Here's how the part is built. I have some questions about the finished solid (model axes, mm). Face numbers are marked on the shaded views. A direction names the side the tool comes from. Give positions to 0.01 mm unless a question says otherwise; leave off trailing zeros. Order: outer loops, then holes, each group sorted by start corner. A loop starts at its lowest first (then second) coordinate and runs counter-clockwise, first axis right, second up.
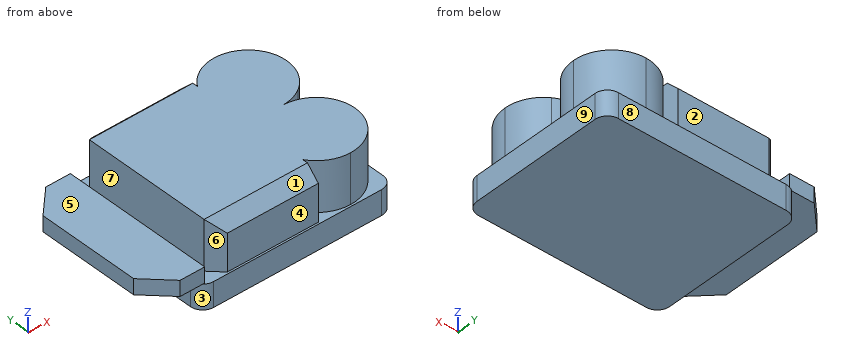
from build123d import *

# Parameters (mm, degrees)
SKETCH_1_W            = 1
SKETCH_1_H            = 2
EXTRUDE_1_DEPTH       = 8
SKETCH_2_W            = 31.3
SKETCH_2_H            = 25.6
EXTRUDE_12_DEPTH      = 4
EXTRUDE_13_DEPTH      = 7
EXTRUDE_13_DEPTH_BACK = 1
SKETCH_3_W            = 2.5
SKETCH_3_H            = 24.6
CHAMFER_1_SIZE        = 4
FILLET_1_R            = 2
CHAMFER_2_SIZE        = 2


with BuildPart() as part:
    # 草图1 → 凸台-拉伸1 (new body)
    with BuildSketch(Plane.XY):
        Polygon((0, 25), (0, 0), (15.8, 0), (15.8, 6.250000037), (15.8, 11.5), (15.8, 13.5), (15.8, 18.749999979), (15.8, 25), align=None)
        with BuildLine():
            Line((16.8, 25), (15.8, 25))
            Line((15.8, 25), (15.8, 18.749999979))
            ThreePointArc((15.8, 18.749999979), (16.055210593, 20.517766943), (16.8, 22.141164992))
            Line((16.8, 22.141164992), (16.8, 25))
        make_face()
        with BuildLine():
            ThreePointArc((16.8, 22.141164992), (16.055210593, 20.517766943), (15.8, 18.749999979))
            ThreePointArc((15.8, 18.749999979), (16.055210599, 16.982233037), (16.8, 15.358835008))
            Line((16.8, 15.358835008), (16.8, 22.141164992))
        make_face()
        with BuildLine():
            ThreePointArc((16.8, 15.358835008), (16.055210599, 16.982233037), (15.8, 18.749999979))
            Line((15.8, 18.749999979), (15.8, 13.5))
            Line((15.8, 13.5), (16.8, 13.5))
            Line((16.8, 13.5), (16.8, 15.358835008))
        make_face()
        with BuildLine():
            ThreePointArc((28.3, 18.75), (26.469417382, 23.169417382), (22.05, 25))
            ThreePointArc((22.05, 25), (19.061043761, 24.238956239), (16.8, 22.141164992))
            Line((16.8, 22.141164992), (16.8, 15.358835008))
            ThreePointArc((16.8, 15.358835008), (17.630582618, 14.330582618), (18.658835008, 13.5))
            Line((18.658835008, 13.5), (25.441164992, 13.5))
            ThreePointArc((25.441164992, 13.5), (27.538956239, 15.761043761), (28.3, 18.75))
        make_face()
        with BuildLine():
            ThreePointArc((18.658835008, 13.5), (17.630582618, 14.330582618), (16.8, 15.358835008))
            Line((16.8, 15.358835008), (16.8, 13.5))
            Line((16.8, 13.5), (18.658835008, 13.5))
        make_face()
        with BuildLine():
            ThreePointArc((16.8, 2.858835008), (19.061043761, 0.761043761), (22.05, 0))
            ThreePointArc((22.05, 0), (26.469417382, 1.830582618), (28.3, 6.25))
            ThreePointArc((28.3, 6.25), (27.538956239, 9.238956239), (25.441164992, 11.5))
            Line((25.441164992, 11.5), (18.658835008, 11.5))
            ThreePointArc((18.658835008, 11.5), (17.630582618, 10.669417382), (16.8, 9.641164992))
            Line((16.8, 9.641164992), (16.8, 2.858835008))
        make_face()
        with BuildLine():
            Line((16.8, 11.5), (16.8, 9.641164992))
            ThreePointArc((16.8, 9.641164992), (17.630582618, 10.669417382), (18.658835008, 11.5))
            Line((18.658835008, 11.5), (16.8, 11.5))
        make_face()
        with BuildLine():
            Line((16.8, 13.5), (16.8, 11.5))
            Line((16.8, 11.5), (18.658835008, 11.5))
            ThreePointArc((18.658835008, 11.5), (20.282233047, 12.244789404), (22.05, 12.5))
            ThreePointArc((22.05, 12.5), (20.282233047, 12.755210596), (18.658835008, 13.5))
            Line((18.658835008, 13.5), (16.8, 13.5))
        make_face()
        with Locations((16.3, 12.5)):
            Rectangle(SKETCH_1_W, SKETCH_1_H)
        with BuildLine():
            ThreePointArc((16.8, 9.641164992), (16.055210601, 8.017766971), (15.8, 6.250000037))
            ThreePointArc((15.8, 6.250000037), (16.055210591, 4.482233065), (16.8, 2.858835008))
            Line((16.8, 2.858835008), (16.8, 9.641164992))
        make_face()
        with BuildLine():
            Line((15.8, 11.5), (15.8, 6.250000037))
            ThreePointArc((15.8, 6.250000037), (16.055210601, 8.017766971), (16.8, 9.641164992))
            Line((16.8, 9.641164992), (16.8, 11.5))
            Line((16.8, 11.5), (15.8, 11.5))
        make_face()
        with BuildLine():
            Line((15.8, 6.250000037), (15.8, 0))
            Line((15.8, 0), (16.8, 0))
            Line((16.8, 0), (16.8, 2.858835008))
            ThreePointArc((16.8, 2.858835008), (16.055210591, 4.482233065), (15.8, 6.250000037))
        make_face()
        with BuildLine():
            ThreePointArc((22.05, 12.5), (20.282233047, 12.244789404), (18.658835008, 11.5))
            Line((18.658835008, 11.5), (25.441164992, 11.5))
            ThreePointArc((25.441164992, 11.5), (23.817766953, 12.244789404), (22.05, 12.5))
        make_face()
        with BuildLine():
            ThreePointArc((18.658835008, 13.5), (20.282233047, 12.755210596), (22.05, 12.5))
            ThreePointArc((22.05, 12.5), (23.817766953, 12.755210596), (25.441164992, 13.5))
            Line((25.441164992, 13.5), (18.658835008, 13.5))
        make_face()
    extrude(amount=EXTRUDE_1_DEPTH)

    # 草图2 → 凸台-拉伸12 (add)
    with BuildSketch(Plane(origin=(0, 0, 0), x_dir=(-1, 0, 0), z_dir=(0, 0, -1))):
        with Locations((-13.15, 12.5)):
            Rectangle(SKETCH_2_W, SKETCH_2_H)
    extrude(amount=EXTRUDE_12_DEPTH)

    # 草图3 → 凸台-拉伸13 (add, two sides: drawn at the far end of the back side and taken through both)
    with BuildSketch(Plane.ZY.offset(2.5).offset(-EXTRUDE_13_DEPTH_BACK)):
        with Locations((1.25, 12.5)):
            Rectangle(SKETCH_3_W, SKETCH_3_H)
    extrude(amount=EXTRUDE_13_DEPTH + EXTRUDE_13_DEPTH_BACK)

    # 倒角1
    chamfer_1_edges = [part.edges().sort_by_distance(p)[0] for p in [
        (-9.5, 0.2, 1.25),
        (-9.5, 24.8, 1.25),
    ]]
    chamfer(chamfer_1_edges, length=CHAMFER_1_SIZE)

    # 圆角1
    # the kernel refuses this fillet: 2 mm, written as the material it takes off along each edge
    with BuildSketch(Plane(origin=(-2.5, -0.3, 0), x_dir=(0, 1, 0), z_dir=(0, 0, -1))) as fillet_1_piece_1:
        with BuildLine():
            CenterArc((FILLET_1_R, FILLET_1_R), FILLET_1_R, 180, 90)
            Line((0, FILLET_1_R), (0, 0))
            Line((0, 0), (FILLET_1_R, 0))
        make_face()
    extrude(amount=9, mode=Mode.SUBTRACT)
    with BuildSketch(Plane(origin=(-2.5, 25.3, 0), x_dir=(0, -1, 0), z_dir=(0, 0, -1))) as fillet_1_piece_2:
        with BuildLine():
            CenterArc((FILLET_1_R, -FILLET_1_R), FILLET_1_R, 90, 90)
            Line((0, -FILLET_1_R), (0, 0))
            Line((0, 0), (FILLET_1_R, 0))
        make_face()
    extrude(amount=9, mode=Mode.SUBTRACT)
    with BuildSketch(Plane(origin=(28.8, 25.3, 5), x_dir=(-1, 0, 0), z_dir=(0, 0, -1))) as fillet_1_piece_3:
        with BuildLine():
            CenterArc((FILLET_1_R, -FILLET_1_R), FILLET_1_R, 90, 90)
            Line((0, -FILLET_1_R), (0, 0))
            Line((0, 0), (FILLET_1_R, 0))
        make_face()
    extrude(amount=14, mode=Mode.SUBTRACT)
    with BuildSketch(Plane(origin=(28.8, -0.3, 5), x_dir=(-1, 0, 0), z_dir=(0, 0, -1))) as fillet_1_piece_4:
        with BuildLine():
            CenterArc((FILLET_1_R, FILLET_1_R), FILLET_1_R, 180, 90)
            Line((0, FILLET_1_R), (0, 0))
            Line((0, 0), (FILLET_1_R, 0))
        make_face()
    extrude(amount=14, mode=Mode.SUBTRACT)

    # 倒角2
    chamfer_2_edges = [part.edges().sort_by_distance(p)[0] for p in [
        (0, 0, 4),
        (0, 25, 4),
        (8.4, 25, 8),
        (8.4, 0, 8),
    ]]
    chamfer(chamfer_2_edges, length=CHAMFER_2_SIZE)


solid = part.part
Q1. If we section it at A-A on z = 0.75: List the corners of the cut face in (x, y) for me.
Filled sheet:
outline: (-9.5, 4.2) - (-5.5, 0.2) - (-1.5, 0.2) - (-1.5, 24.8) - (-5.5, 24.8) - (-9.5, 20.8) - close; (0, 2) - (2, 0) - (16.8, 0) - (16.8, 2.86) arc R6.25 ccw (long way) to (22.05, 12.5) arc R6.25 ccw (long way) to (16.8, 22.14) - (16.8, 25) - (2, 25) - (0, 23) - close
Q2. I need wall thicknesses on L1, parallel to X at y = 10.25, z = -1; L2, parallel to X at y = 22.5, z = 7.75; L3, parallel to X at y = 13.5, z = 0.75. Which ranges of each line are inside material? Lowest first, please.
Filled sheet:
L1: x = -2.5 to 28.8
L2: x = 0 to 16.8, 17.05 to 27.05
L3: x = -9.5 to -1.5, 0 to 25.44
Q3. If we section it at D-D on y = 5.75: List the corners of the cut face in (x, z) for me.
Filled sheet:
outline: (-9.5, 0) - (-2.5, 0) - (-2.5, -4) - (28.8, -4) - (28.8, 0) - (28.28, 0) - (28.28, 8) - (0, 8) - (0, 0) - (-1.5, 0) - (-1.5, 2.5) - (-9.5, 2.5) - close
Q4. If we section it at B-B on x = 6.5: List the corners of the cut face in (y, z) for me, plus the area to 3 significant figures.
Filled sheet:
outline: (-0.3, -4) - (25.3, -4) - (25.3, 0) - (25, 0) - (25, 6) - (23, 8) - (2, 8) - (0, 6) - (0, 0) - (-0.3, 0) - close
area: 298 mm2
Q5. I'm going to push flat-ended pins straight in: P1, Ø1.5, axis at y = 13, z = 3.5, coming from the +X side; P2, Ø2, axis at x = -2.5, z = 1, coming from the +Y side; P3, Ø2.5, axis at x = -5, y = 11, coming from the +Z side. Where does each tip first touch, or does it pass through?
Filled sheet:
P1: stops at x = 25.8
P2: stops at y = 24.8
P3: stops at z = 2.5
Q6. Thinking about a two-plate mould opening in X: for the marked faces 6, 7, 8 and 9, which applies, released by +X, released by -X, zero draft, split by the parting line, or undercut?
Filled sheet:
face 6: undercut
face 7: undercut
face 8: zero draft
face 9: released by +X
Q7. If we section it at C-C on z = 3.5: List the corners of the cut face in (x, y) for me, plus the area to 3 significant figures.
Filled sheet:
outline: (0, 2) - (2, 0) - (16.8, 0) - (16.8, 2.86) arc R6.25 ccw (long way) to (22.05, 12.5) arc R6.25 ccw (long way) to (16.8, 22.14) - (16.8, 25) - (2, 25) - (0, 23) - close
area: 661 mm2
Q8. For the marked faces 1, 2, 3, 4 and 5, which set-ups out of +Z, -Z, +X, -X, +Y, -Y let a thin tool reach every point of the face, with its end or its side?
Filled sheet:
face 1: +Z, -X, -Y
face 2: +Z, +X, -X, +Y
face 3: -Z, -X, -Y
face 4: +Z, +X, -X, -Y
face 5: +Z, -X, +Y, -Y
